from build123d import *

# Parameters (mm, degrees)
SKETCH1_W                         = 254
SKETCH1_H                         = 304.8
BOSS_EXTRUDE1_DEPTH               = 25.4
F_10_0_10_DIAMETER_HOLE1_D        = 10
TAP_DRILL_FOR_M12X1_75_TAP1_D     = 10.2
TAP_DRILL_FOR_M12X1_75_TAP1_DEPTH = 30
TAP_DRILL_FOR_M12X1_75_TAP1_TIP   = 3.064389157


with BuildPart() as part:
    # Sketch1 → Boss-Extrude1 (new body)
    with BuildSketch(Plane.XY):
        Rectangle(SKETCH1_W, SKETCH1_H)
    extrude(amount=BOSS_EXTRUDE1_DEPTH)

    # Ø10.0 (10) Diameter Hole1 (through all)
    with Locations(Plane.XY.offset(25.4)):
        with Locations((-114.3, -139.7), (0, -139.7), (114.3, -139.7)):
            Hole(F_10_0_10_DIAMETER_HOLE1_D / 2)

    # Tap Drill for M12x1.75 Tap1
    with Locations(Plane(origin=(0, 152.4, 0), x_dir=(1, 0, 0), z_dir=(0, 1, 0))):
        with Locations((-47.754, -12.7), (47.498, -12.7)):
            Hole(TAP_DRILL_FOR_M12X1_75_TAP1_D / 2, depth=TAP_DRILL_FOR_M12X1_75_TAP1_DEPTH)
            with Locations((0, 0, -(TAP_DRILL_FOR_M12X1_75_TAP1_DEPTH + TAP_DRILL_FOR_M12X1_75_TAP1_TIP / 2))):  # 118° drill point
                Cone(0, TAP_DRILL_FOR_M12X1_75_TAP1_D / 2, TAP_DRILL_FOR_M12X1_75_TAP1_TIP, mode=Mode.SUBTRACT)


solid = part.part
Geometry: final body of the model. Coordinates: model frame, mm. A direction names the side the tool comes from. Give positions to 0.01 mm unless a question says otherwise; leave off trailing zeros. Write each loop counter-clockwise with the first axis right and the second up, starting at its lowest first coordinate (ties: lowest second). Pieces come first, ordered by that corner, then holes. Notation, with made-up numbers: (-22.75, 14.5) - (-1.75, 14.5) arc R26 cw to (-1.75, 40.5) - close; hole circle Ø3 at (61, 77.5). An arc over 180 degrees is marked (long way). Return JSON: item names as keys, results as strings. Group by question number.
1) Set-up query: faces 1 (the cylindrical face through (-42.66, 137.19, 12.48)), 2 (the cylindrical face through (-113.22, -144.58, 12.52)). Return all of +Z, -Z, +X, -X, +Y, -Y with unobstructed straight access to the full face (end or side cutting, diameter ignored); none if empty.
2) First-contact query: P1, Ø6, axis at x = 47.498, z = 12.7, coming from the +Y side. Flat tip, straight axial feed; report the tip coordinate or a pass-through.
3) Section B-B on x = 0. Return the cut outline in (y, z).
4) Mould query, pull axis Z, two halves, no side actions, for faces 3 (the flat face through (-127, -2, 13)), 4 (the cylindrical face through (51.55, 137.19, 15.8)), 5 (the conical face through (46.61, 119.87, 12.66)), 6 (the flat face through (-2, 2, 25.4)). Classes: released by +Z, released by -Z, zero draft, split by the parting line, or undercut.
5) Section A-A on y = -139.7. Return the cut outline in (x, z), plus the area to 3 significant figures.
6) Line query: line 1 (Y direction, x = -114.3, z = 13.75); line 2 (Y direction, x = -3.5, z = 12.5). Output: solid intervals per line, ascending.
Filled in:
{
 "1": {"face 1": "+Y", "face 2": "+Z, -Z"},
 "2": {"P1": "stops at y = 121.14"},
 "3": {"outline": "(-152.4, 0) - (-144.7, 0) - (-144.7, 25.4) - (-152.4, 25.4) - close; (-134.7, 0) - (152.4, 0) - (152.4, 25.4) - (-134.7, 25.4) - close"},
 "4": {"face 3": "zero draft", "face 4": "undercut", "face 5": "undercut", "face 6": "released by +Z"},
 "5": {"outline": "(-127, 0) - (-119.3, 0) - (-119.3, 25.4) - (-127, 25.4) - close; (-109.3, 0) - (-5, 0) - (-5, 25.4) - (-109.3, 25.4) - close; (5, 0) - (109.3, 0) - (109.3, 25.4) - (5, 25.4) - close; (119.3, 0) - (127, 0) - (127, 25.4) - (119.3, 25.4) - close", "area": "5,690 mm^2"},
 "6": {"line 1": "y = -152.4 to -144.7, -134.7 to 152.4", "line 2": "y = -152.4 to -143.27, -136.13 to 152.4"}
}
